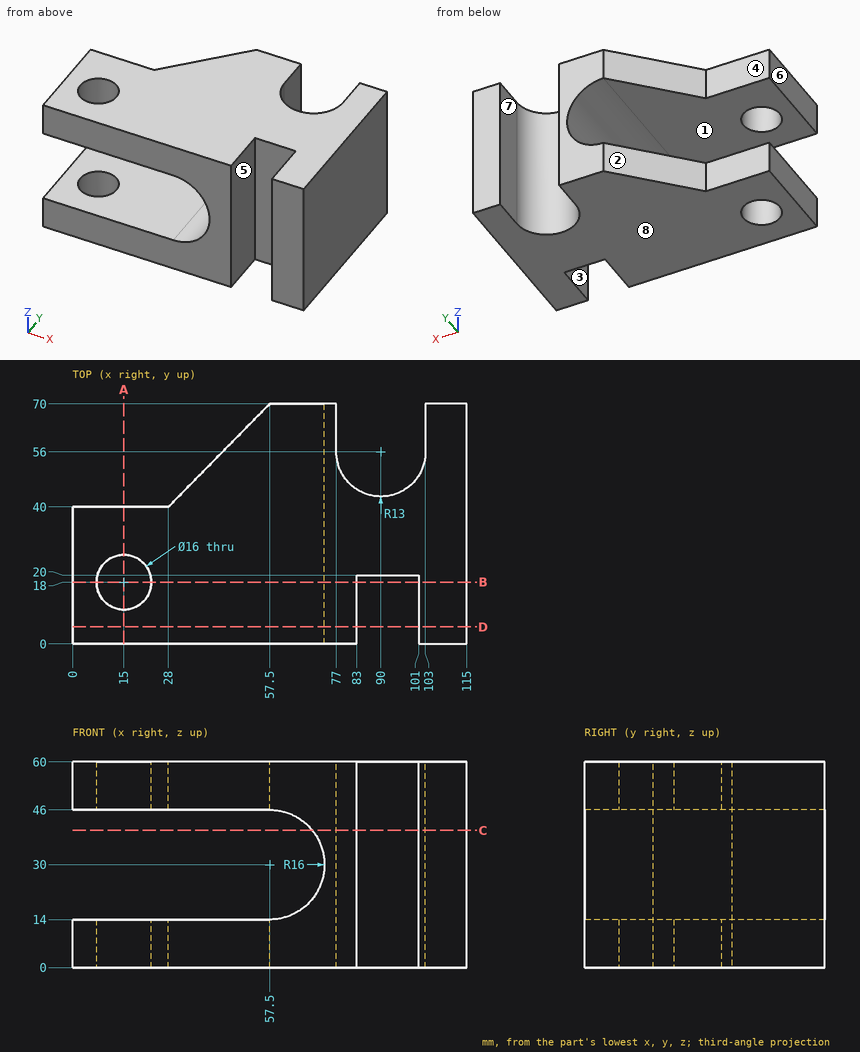
Check sheet for the drawn part. Datum: minimum x, y, z corner. Units: mm. A direction names the side the tool comes from. Round coordinates to 2 decimals unless told otherwise and drop trailing zeros. Write each loop counter-clockwise with the first axis right and the second up, starting at its lowest first coordinate (ties: lowest second). Pieces come first, ordered by that corner, then holes. Notation, with made-up numbers: (28, 12) -> (75, 12) arc R16 cw to (75, 41) -> close; hole circle Ø11 at (28.5, 54). An arc over 180 degrees is marked (long way). Write each question's results on one line, items separated by ' | '. Start each with the question number.
1. Cross-section at B-B (y = 18). Enter the section's corners in (x, z), then the cut area to 3 significant figures.
2. Cross-section at D-D (y = 5). Enter the section's corners in (x, z).
3. Cross-section at C-C (z = 40). Enter the section's corners in (x, y), then the cut area to 3 significant figures.
4. Cross-section at A-A (x = 15). Enter the section's corners in (y, z).
5. Material ranges on probe 1 along X at (y, z) = (18, 5); probe 2 along Z at (x, y) = (52.5, 48); probe 3 along Y at (x, z) = (15, 56), recorded low to high. Write a range as from..to.
6. Depth check by flat-ended pin: P1, Ø9, axis at x = 92, z = 17.5, coming from the -Y side; P2, Ø6, axis at y = 11, z = 28.5, coming from the -X side; P3, Ø15.5, axis at x = 7.5, z = 9, coming from the +Y side. Enter the tip coordinate at first touch or a pass-through.
7. Set-up check for the marked faces 4, 5, 6, 7 and 8: record each of +Z, -Z, +X, -X, +Y, -Y from which the full face is reachable in a straight line by a thin tool's end or side.
8. Draft check along X on the marked faces 1, 2 and 3. Enter one of: +X half, -X half, draft (parallel to the pull), parting line (faces both ways), or undercut.
Solutions:
1) outline: (0, 0) -> (7, 0) -> (7, 14) -> (0, 14) -> close; (0, 46) -> (7, 46) -> (7, 60) -> (0, 60) -> close; (23, 0) -> (83, 0) -> (83, 60) -> (23, 60) -> (23, 46) -> (57.5, 46) arc R16 cw to (57.5, 14) -> (23, 14) -> close; (101, 0) -> (115, 0) -> (115, 60) -> (101, 60) -> close | area: 3,130 mm2
2) outline: (0, 0) -> (83, 0) -> (83, 60) -> (0, 60) -> (0, 46) -> (57.5, 46) arc R16 cw to (57.5, 14) -> (0, 14) -> close; (101, 0) -> (115, 0) -> (115, 60) -> (101, 60) -> close
3) outline: (69.99, 0) -> (83, 0) -> (83, 20) -> (101, 20) -> (101, 0) -> (115, 0) -> (115, 70) -> (103, 70) -> (103, 56) arc R13 cw to (77, 56) -> (77, 70) -> (69.99, 70) -> close | area: 2,160 mm2
4) outline: (0, 0) -> (10, 0) -> (10, 14) -> (0, 14) -> close; (0, 46) -> (10, 46) -> (10, 60) -> (0, 60) -> close; (26, 0) -> (40, 0) -> (40, 14) -> (26, 14) -> close; (26, 46) -> (40, 46) -> (40, 60) -> (26, 60) -> close
5) probe 1: x = 0..7, 23..83, 101..115 | probe 2: z = 0..14, 46..60 | probe 3: y = 0..10, 26..40
6) P1: stops at y = 20 | P2: stops at x = 72.85 | P3: stops at y = 40
7) face 4: +Z, -Z, -X, +Y | face 5: +Z, -Z, -Y | face 6: +Z, -Z, -X, +Y, -Y | face 7: +Z, -Z, +Y | face 8: -Z, +X, -X, +Y, -Y
8) face 1: draft | face 2: -X half | face 3: undercut
